from build123d import *

# Parameters (mm, degrees)
SKETCH1_W           = 45
SKETCH1_H           = 20
BOSS_EXTRUDE1_DEPTH = 4
SKETCH2_W           = 10
SKETCH2_H           = 10
BOSS_EXTRUDE2_DEPTH = 2
SKETCH3_R           = 8.5
BOSS_EXTRUDE3_DEPTH = 12
BOSS_EXTRUDE4_DEPTH = 3


with BuildPart() as part:
    # Sketch1 → Boss-Extrude1 (new body)
    with BuildSketch(Plane.XY):
        Rectangle(SKETCH1_W, SKETCH1_H)
    extrude(amount=BOSS_EXTRUDE1_DEPTH)

    # Sketch2 → Boss-Extrude2 (add)
    with BuildSketch(Plane(origin=(0, 0, 0), x_dir=(-1, 0, 0), z_dir=(0, 0, -1))):
        with Locations((0, 12.5)):
            Rectangle(SKETCH2_W, SKETCH2_H)
    extrude(amount=BOSS_EXTRUDE2_DEPTH)

    # Sketch3 → Boss-Extrude3 (add)
    with BuildSketch(Plane.XY.offset(4)):
        with Locations((-13, 0)):
            Circle(SKETCH3_R)
        with Locations(Location((13, 0, 0), (0, 0, 180))):
            Circle(SKETCH3_R)
    extrude(amount=BOSS_EXTRUDE3_DEPTH)

    # Sketch4 → Boss-Extrude4 (add)
    with BuildSketch(Plane.XY.offset(4)):
        with BuildLine():
            Line((3.5, -9.9), (-3.5, -9.9))
            ThreePointArc((-3.5, -9.9), (-5.9, -7.5), (-3.5, -5.1))
            Line((-3.5, -5.1), (3.5, -5.1))
            ThreePointArc((3.5, -5.1), (5.9, -7.5), (3.5, -9.9))
        make_face()
    extrude(amount=BOSS_EXTRUDE4_DEPTH)


solid = part.part
Work out the finished part from the listing and answer in its coordinate system (mm). A direction names the side the tool comes from. Round coordinates to 2 decimals unless told otherwise and drop trailing zeros. Loops run counter-clockwise (first coordinate to the right, second up) from the corner with the lowest first, then second, coordinate; pieces in that order, holes last. Notation, with made-up numbers: (-19, -35) -> (-12, -35) arc R15 ccw to (-12, -24) -> close; hole circle Ø9 at (-28, -21.5). An arc over 180 degrees is marked (long way). Use one line per item in the form item = value.
(1) Find section B-B on x = -17. Give the vertices of the cut face in (y, z), then the cut area to 3 significant figures.
Answer list:
outline = (-10, 0) -> (10, 0) -> (10, 4) -> (7.5, 4) -> (7.5, 16) -> (-7.5, 16) -> (-7.5, 4) -> (-10, 4) -> close
area = 260 mm2
(2) Flat-ended cylindrical pins translate along their axes: P1, Ø1, axis at y = 13, z = -1, coming from the -X side; P2, Ø1, axis at x = -2, z = -1, coming from the -Y side; P3, Ø1.2, axis at x = 6, z = 2, coming from the +Y side. Find the tip coordinate at first contact, or state that the pin passes through.
Answer list:
P1 = -5
P2 = 7.5
P3 = 10
(3) For a pull along X with two mould halves and no side action, classify faces 6 (the flat face through (22.5, 0, 2)), 7 (the flat face through (0, 14, 0)), 8 (the cylindrical face through (-19.265, 5.745, 9.916)) as released by +X, released by -X, zero draft, split by the parting line, or undercut.
Answer list:
face_6 = released by +X
face_7 = zero draft
face_8 = undercut
(4) Find section A-A on y = 0. Give the vertices of the cut face in (x, z), then the cut area to 3 significant figures.
Answer list:
outline = (-22.5, 0) -> (22.5, 0) -> (22.5, 4) -> (21.5, 4) -> (21.5, 16) -> (4.5, 16) -> (4.5, 4) -> (-4.5, 4) -> (-4.5, 16) -> (-21.5, 16) -> (-21.5, 4) -> (-22.5, 4) -> close
area = 588 mm2
(5) Find section D-D on y = -7.5. Give the vertices of the cut face in (x, z).
Answer list:
outline = (-22.5, 0) -> (22.5, 0) -> (22.5, 4) -> (17, 4) -> (17, 16) -> (9, 16) -> (9, 4) -> (5.9, 4) -> (5.9, 7) -> (-5.9, 7) -> (-5.9, 4) -> (-9, 4) -> (-9, 16) -> (-17, 16) -> (-17, 4) -> (-22.5, 4) -> close
(6) Find section C-C on z = 11.75. Give the vertices of the cut face in (x, y), then the cut area to 3 significant figures.
Answer list:
outline = circle Ø17 at (-13, 0); circle Ø17 at (13, 0)
area = 454 mm2
(7) A tool of negligible diameter and unlimited length cuts with its end or side. For faces 1 (the flat face through (5, 12, -1)), 2 (the cylindrical face through (5.9, -7.45, 5.48)), 3 (the flat face through (0, 7.5, -1)), 4 (the flat face through (0, -5.1, 5)), 5 (the flat face through (0, -7, 7)), from which of +Z, -Z, +X, -X, +Y, -Y can it reach the whole face along a straight path? Write none if from no direction.
Answer list:
face_1 = -Z, +X, +Y, -Y
face_2 = +Z
face_3 = -Z, +X, -X, -Y
face_4 = +Z, +Y
face_5 = +Z, -Y
(8) Straight lines are drawn through the part: line 1 (Z direction, x = -11.5, y = 1.75); line 2 (Y direction, x = 12.5, z = 0.75); line 3 (Z direction, x = 6.5, y = -6.25). For each, find the intervals that lie inside material, in ascending order.
Answer list:
line_1 = 0 to 16
line_2 = -10 to 10
line_3 = 0 to 4
